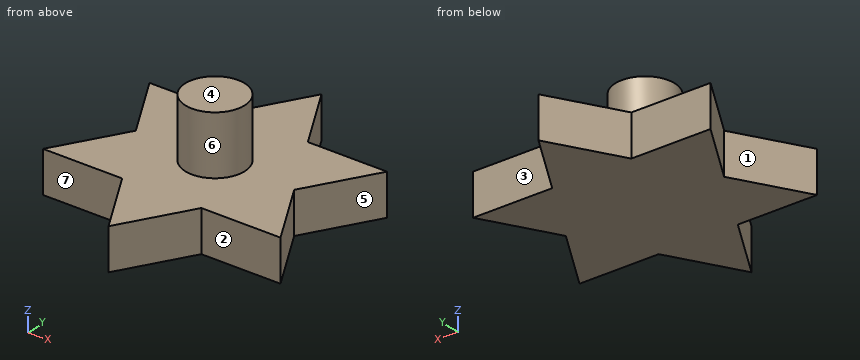
```python
from build123d import *

# Parameters (mm, degrees)
BOSS_EXTRU_1_DEPTH = 7
ESQUISSE2_R        = 5
BOSS_EXTRU_2_DEPTH = 10


with BuildPart() as part:
    # Esquisse1 → Boss.-Extru.1 (new body)
    with BuildSketch(Plane.XY):
        Polygon((-20, 11.547005384), (-6.666666667, 11.547005384), (0, 23.094010768), (6.666666667, 11.547005384), (20, 11.547005384), (13.333333333, 0), (20, -11.547005384), (6.666666667, -11.547005384), (0, -23.094010768), (-6.666666667, -11.547005384), (-20, -11.547005384), (-13.333333333, 0), align=None)
    extrude(amount=BOSS_EXTRU_1_DEPTH)

    # Esquisse2 → Boss.-Extru.2 (add)
    with BuildSketch(Plane.XY.offset(7)):
        Circle(ESQUISSE2_R)
    extrude(amount=BOSS_EXTRU_2_DEPTH)


solid = part.part
```
Input: part model. Units: mm. Frame: model coordinates. Face numbers are marked on the shaded views. A direction names the side the tool comes from. Coordinates: 2 decimals unless noted, no trailing zeros. Write each loop counter-clockwise with the first axis right and the second up, starting at its lowest first coordinate (ties: lowest second). Pieces come first, ordered by that corner, then holes.
1) Pin query (flat end, axial travel): pin 1 Ø3.5 at (x, z) = (10, 4.5) entering from +Y; pin 2 Ø7.5 at (x, z) = (-13, 2) entering from -Y. Return the tip coordinate at first contact, or that it passes through.
2) Section D-D on x = -1.5. Output: boundary loops of the cut face in (y, z), and give its area (3 significant figures).
3) Section B-B on y = 1. Output: boundary loops of the cut face in (x, z).
4) Material intervals for line 1 along Z through (x, y) = (-2, -13.5); line 2 along Y through (x, z) = (8.5, 6.25); line 3 along Y through (x, z) = (-16, 2), sorted ascending.
5) Section A-A on z = 6. Output: boundary loops of the cut face in (x, y), and give its area (3 significant figures).
6) Mould query, pull axis Y, two halves, no side actions, for the marked faces 4, 5, 6 and 7. Classes: pulls with the +Y half, pulls with the -Y half, needs draft (parallel to the pull), parting line crosses it, or undercut.
7) Set-up query: the marked faces 1, 2 and 3. Return all of +Z, -Z, +X, -X, +Y, -Y with unobstructed straight access to the full face (end or side cutting, diameter ignored); none if empty.
8) Section C-C on x = -9.5. Output: boundary loops of the cut face in (y, z), and give its area (3 significant figures).
Check result:
1. pin 1: stops at y = 11.55
1. pin 2: stops at y = -11.55
2. outline: (-20.5, 0) - (20.5, 0) - (20.5, 7) - (4.77, 7) - (4.77, 17) - (-4.77, 17) - (-4.77, 7) - (-20.5, 7) - close
2. area: 382 mm2
3. outline: (-13.91, 0) - (13.91, 0) - (13.91, 7) - (4.9, 7) - (4.9, 17) - (-4.9, 17) - (-4.9, 7) - (-13.91, 7) - close
4. line 1: z = 0 to 7
4. line 2: y = -11.55 to 11.55
4. line 3: y = -11.55 to -4.62, 4.62 to 11.55
5. outline: (-20, -11.55) - (-6.67, -11.55) - (0, -23.09) - (6.67, -11.55) - (20, -11.55) - (13.33, 0) - (20, 11.55) - (6.67, 11.55) - (0, 23.09) - (-6.67, 11.55) - (-20, 11.55) - (-13.33, 0) - close
5. area: 924 mm2
6. face 4: needs draft
6. face 5: undercut
6. face 6: parting line crosses it
6. face 7: pulls with the -Y half
7. face 1: +Z, -Z, -X
7. face 2: +Z, -Z, +X, -Y
7. face 3: +Z, -Z, +X, +Y
8. outline: (-11.55, 0) - (11.55, 0) - (11.55, 7) - (-11.55, 7) - close
8. area: 162 mm2
